Source: CAD feature listing. Evaluate the final solid. Frame: model axes, mm. A direction names the side the tool comes from. Round coordinates to 2 decimals unless told otherwise and drop trailing zeros. Write each loop counter-clockwise with the first axis right and the second up, starting at its lowest first coordinate (ties: lowest second). Pieces come first, ordered by that corner, then holes.
from build123d import *

# Parameters (mm, degrees)
SKETCH1_W              = 323.6
SKETCH1_H              = 350
BASE_FLANGE1_DEPTH     = 0.8
SKETCHED_START         = -175
SKETCHED_BEND3_DEPTH   = 350
SKETCHED_BEND3_2_DEPTH = 350


# Read off the part's stored shape, not the designer's step: Sketched Bend3
# Sheet-metal steps are written as plain solids
with BuildPart() as part:
    # Sketch1 → Base-Flange1 (new body)
    with BuildSketch(Plane(origin=(0, 0, 0), x_dir=(1, 0, 0), z_dir=(0, 1, 0))):
        Rectangle(SKETCH1_W, SKETCH1_H)
    extrude(amount=BASE_FLANGE1_DEPTH)

    # Sketched Bend3 outline → Sketched Bend3 (cut)
    with BuildSketch(Plane.XY.offset(SKETCHED_START)):
        with BuildLine():
            Line((161.8, 0.8), (-123.802894475, 0.8))
            ThreePointArc((-123.802894475, 0.8), (-124.451029292, 0.212549213), (-125.299557429, 0))
            Line((-125.299557429, 0), (161.8, 0))
            Line((161.8, 0), (161.8, 0.8))
        make_face()
        with BuildLine():
            Line((-161.8, 0), (-151.500442571, 0))
            ThreePointArc((-151.500442571, 0), (-152.348970708, 0.212549213), (-152.997105525, 0.8))
            Line((-152.997105525, 0.8), (-161.8, 0.8))
            Line((-161.8, 0.8), (-161.8, 0))
        make_face()
    extrude(amount=SKETCHED_BEND3_DEPTH, mode=Mode.SUBTRACT)

    # Sketched Bend3 2 outline → Sketched Bend3 2 (add)
    with BuildSketch(Plane.XY.offset(SKETCHED_START)):
        with BuildLine():
            ThreePointArc((-123.802894475, 0.8), (-123.577060213, 1.277502784), (-123.499557429, 1.8))
            Line((-123.499557429, 1.8), (-123.499557429, 248.000885142))
            ThreePointArc((-123.499557429, 248.000885142), (-124.026765223, 249.273677349), (-125.299557429, 249.800885142))
            Line((-125.299557429, 249.800885142), (-151.500442571, 249.800885142))
            ThreePointArc((-151.500442571, 249.800885142), (-152.773234777, 249.273677348), (-153.300442571, 248.000885142))
            Line((-153.300442571, 248.000885142), (-153.300442571, 239.900442571))
            Line((-153.300442571, 239.900442571), (-152.500442571, 239.900442571))
            Line((-152.500442571, 239.900442571), (-152.500442571, 248.000885142))
            ThreePointArc((-152.500442571, 248.000885142), (-152.207549352, 248.707991924), (-151.500442571, 249.000885142))
            Line((-151.500442571, 249.000885142), (-125.299557429, 249.000885142))
            ThreePointArc((-125.299557429, 249.000885142), (-124.592450648, 248.707991924), (-124.299557429, 248.000885142))
            Line((-124.299557429, 248.000885142), (-124.299557429, 1.8))
            ThreePointArc((-124.299557429, 1.8), (-124.592450648, 1.092893219), (-125.299557429, 0.8))
            Line((-125.299557429, 0.8), (-123.802894475, 0.8))
        make_face()
        with BuildLine():
            Line((-152.997105525, 0.8), (-151.500442571, 0.8))
            ThreePointArc((-151.500442571, 0.8), (-152.207549352, 1.092893219), (-152.500442571, 1.8))
            Line((-152.500442571, 1.8), (-152.500442571, 9.900442571))
            Line((-152.500442571, 9.900442571), (-153.300442571, 9.900442571))
            Line((-153.300442571, 9.900442571), (-153.300442571, 1.8))
            ThreePointArc((-153.300442571, 1.8), (-153.222939787, 1.277502784), (-152.997105525, 0.8))
        make_face()
    extrude(amount=SKETCHED_BEND3_2_DEPTH)


solid = part.part
1) Material intervals for line 1 (Y direction, x = -138.5, z = 67.5); line 2 (X direction, y = 186.5, z = 8.5); line 3 (Y direction, x = -124.75, z = -137), sorted ascending.
Taken from the geometry:
line 1: y = 0 to 0.8, 249 to 249.8
line 2: x = -124.3 to -123.5
line 3: y = 0.09 to 0.96, 248.84 to 249.71
2) Contact query for flat-ended pins moving along their axis: P1, Ø10, axis at y = 78, z = 40, coming from the -X side; P2, Ø0.9, axis at x = -152.5, z = -77, coming from the -Y side. Output: stop coordinate, or through.
Taken from the geometry:
P1: stops at x = -124.3
P2: stops at y = 0.09
3) Section query B-B on z = 114.5. Return the cut outline in (x, y).
Taken from the geometry:
outline: (-153.3, 1.8) arc R1.8 ccw to (-151.5, 0) - (-125.3, 0) arc R1.8 ccw to (-123.5, 1.8) - (-123.5, 248) arc R1.8 ccw to (-125.3, 249.8) - (-151.5, 249.8) arc R1.8 ccw to (-153.3, 248) - (-153.3, 239.9) - (-152.5, 239.9) - (-152.5, 248) arc R1 cw to (-151.5, 249) - (-125.3, 249) arc R1 cw to (-124.3, 248) - (-124.3, 1.8) arc R1 cw to (-125.3, 0.8) - (-151.5, 0.8) arc R1 cw to (-152.5, 1.8) - (-152.5, 9.9) - (-153.3, 9.9) - close
4) Reachability of faces 5 (the face through (-152.5, 6, -2)), 6 (the face through (-138, 249.801, -2)) from +Z, -Z, +X, -X, +Y, -Y: full face, straight path, thin tool, end or side. Return the list, or none.
Taken from the geometry:
face 5: +Z, -Z
face 6: +Z, -Z, +X, -X, +Y
5) Pull-direction query (X, two-part tool) for faces 1 (the face through (-123.5, 123, -2)), 2 (the face through (-124, 125, 175)), 3 (the face through (-153.3, 6, -2)), 4 (the face through (-139, 0.8, -2)); classes: released by +X, released by -X, zero draft, split by the parting line, or undercut.
Taken from the geometry:
face 1: released by +X
face 2: zero draft
face 3: released by -X
face 4: undercut
6) Section query C-C on y = 152. Return the cut outline in (x, z), then the cut area to 3 significant figures.
Taken from the geometry:
outline: (-124.3, -175) - (-123.5, -175) - (-123.5, 175) - (-124.3, 175) - close
area: 280 mm2
7) Section query A-A on x = -145. Return the cut outline in (y, z), then the cut area to 3 significant figures.
Taken from the geometry:
outline: (0, -175) - (0.8, -175) - (0.8, 175) - (0, 175) - close; (249, -175) - (249.8, -175) - (249.8, 175) - (249, 175) - close
area: 560 mm2
